from build123d import *

# Parameters (mm, degrees)
F0_W     = 53
F0_H     = 37
F1_DEPTH = 1.6
F2_W     = 8
F2_H     = 30.5
F3_DEPTH = 10
F4_R     = 1.8
F5_DEPTH = 1.6


with BuildPart() as f1:
    # F0 (on Top) → F1 (new body)
    with BuildSketch(Plane.XY):
        Rectangle(F0_W, F0_H)
    extrude(amount=F1_DEPTH)

    # F2 (on face) → F3 (join)
    with BuildSketch(Plane.XY.offset(1.6)):
        with Locations((21.5, 0)):
            Rectangle(F2_W, F2_H)
        with Locations((-21.5, 0)):
            Rectangle(F2_W, F2_H)
    extrude(amount=F3_DEPTH)

    # F4 (on face) → F5 (cut, through all)
    with BuildSketch(Plane.XY.offset(1.6)):
        with Locations((12.5, -15)):
            Circle(F4_R)
        with Locations((12.5, 15)):
            Circle(F4_R)
        with Locations((-12.5, 15)):
            Circle(F4_R)
        with Locations((-12.5, -15)):
            Circle(F4_R)
    extrude(amount=-F5_DEPTH, mode=Mode.SUBTRACT)


solid = f1.part
Source: CAD feature listing. Evaluate the final solid. Frame: model axes, mm. A direction names the side the tool comes from. Coordinates: 2 decimals unless noted, no trailing zeros. Loops run counter-clockwise (first coordinate to the right, second up) from the corner with the lowest first, then second, coordinate; pieces in that order, holes last. Notation, with made-up numbers: (-29.75, 70) - (25.25, 70) arc R17 cw to (25.25, 97) - close; hole circle Ø6 at (21, 55). An arc over 180 degrees is marked (long way). Return JSON: item names as keys, results as strings.
Q1. Access query for faces 4 (the flat face through (17.5, 0, 7)), 5 (the flat face through (25.5, 0, 7)), 6 (the flat face through (21, -15.25, 7)), 7 (the flat face through (0, 0, 0)), 8 (the flat face through (-25.5, 0, 7)). Directions: +Z, -Z, +X, -X, +Y, -Y. A direction counts if a zero-diameter tool reaches every point of the face in a straight line with its end or side. Return the directions, or none.
Results:
{"face 4": "+Z, +Y, -Y", "face 5": "+Z, +X, +Y, -Y", "face 6": "+Z, +X, -X, -Y", "face 7": "-Z, +X, -X, +Y, -Y", "face 8": "+Z, -X, +Y, -Y"}
Q2. Contact query for flat-ended pins moving along their axis: P1, Ø3, axis at x = -12.5, y = -15, coming from the +Z side; P2, Ø3, axis at y = -6, z = 9, coming from the -X side; P3, Ø3, axis at y = 5.5, z = 8.5, coming from the +X side; P4, Ø4, axis at x = -12.5, y = -10, coming from the +Z side. Output: stop coordinate, or through.
Results:
{"P1": "through", "P2": "x = -25.5", "P3": "x = 25.5", "P4": "z = 1.6"}
Q3. Material intervals for line 1 along Y through (x, z) = (12.5, 0.4); line 2 along X through (y, z) = (10, 3.25); line 3 along Z through (x, y) = (-10.5, -7), sorted ascending.
Results:
{"line 1": "-18.5 to -16.8, -13.2 to 13.2, 16.8 to 18.5", "line 2": "-25.5 to -17.5, 17.5 to 25.5", "line 3": "0 to 1.6"}
Q4. Mould query, pull axis Y, two halves, no side actions, for faces 1 (the flat face through (21, 15.25, 7)), 2 (the flat face through (-26.5, 0, 1)), 3 (the cylindrical face through (-12.734, -13.215, 0.811)). Classes: released by +Y, released by -Y, zero draft, split by the parting line, or undercut.
Results:
{"face 1": "released by +Y", "face 2": "zero draft", "face 3": "undercut"}
Q5. Section C-C, the plane y = -5. Return loops of the section in (x, z), plus the area to 3 significant figures.
Results:
{"outline": "(-26.5, 0) - (26.5, 0) - (26.5, 1.6) - (25.5, 1.6) - (25.5, 11.6) - (17.5, 11.6) - (17.5, 1.6) - (-17.5, 1.6) - (-17.5, 11.6) - (-25.5, 11.6) - (-25.5, 1.6) - (-26.5, 1.6) - close", "area": "245 mm2"}
Q6. Section A-A, the plane z = 9.75. Return loops of the section in (x, y), plus the area to 3 significant figures.
Results:
{"outline": "(-25.5, -15.25) - (-17.5, -15.25) - (-17.5, 15.25) - (-25.5, 15.25) - close; (17.5, -15.25) - (25.5, -15.25) - (25.5, 15.25) - (17.5, 15.25) - close", "area": "488 mm2"}
Q7. Section B-B, the plane x = 12.5. Return loops of the section in (y, z), plus the area to 3 significant figures.
Results:
{"outline": "(-18.5, 0) - (-16.8, 0) - (-16.8, 1.6) - (-18.5, 1.6) - close; (-13.2, 0) - (13.2, 0) - (13.2, 1.6) - (-13.2, 1.6) - close; (16.8, 0) - (18.5, 0) - (18.5, 1.6) - (16.8, 1.6) - close", "area": "47.7 mm2"}
Q8. Section D-D, the plane x = -18.5. Return loops of the section in (y, z), plus the area to 3 significant figures.
Results:
{"outline": "(-18.5, 0) - (18.5, 0) - (18.5, 1.6) - (15.25, 1.6) - (15.25, 11.6) - (-15.25, 11.6) - (-15.25, 1.6) - (-18.5, 1.6) - close", "area": "364 mm2"}
